Verification items for the finished model (mm, model axes). Face numbers are marked on the shaded views. A direction names the side the tool comes from. Round coordinates to 2 decimals unless told otherwise and drop trailing zeros. Loops run counter-clockwise (first coordinate to the right, second up) from the corner with the lowest first, then second, coordinate; pieces in that order, holes last. Notation, with made-up numbers: M 59.25,6.25 L 66.25,6.25 A17 ccw 66.25,32.25 Z; hole C -31,29 d6. An arc over 180 degrees is marked long. Answer as CSV lines item,"result".
```python
from build123d import *

# Parameters (mm, degrees)
F0_W     = 69
F0_H     = 20
F1_DEPTH = 24
F2_W     = 65
F2_H     = 20
F3_DEPTH = 20
F5_W     = 5
F5_H     = 11
F6_DEPTH = 5


with BuildPart() as f1:
    # F0 (on Front) → F1 (new body)
    with BuildSketch(Plane.XZ):
        with Locations((34.5, -10)):
            Rectangle(F0_W, F0_H)
    extrude(amount=F1_DEPTH)

    # F2 (on Top) → F3 (cut, symmetric)
    with BuildSketch(Plane.XY):
        with Locations((34.5, -12)):
            Rectangle(F2_W, F2_H)
    extrude(amount=F3_DEPTH, both=True, mode=Mode.SUBTRACT)

    # F5 (on offset) → F6 (cut)
    with BuildSketch(Plane(origin=(0, -22, 0), x_dir=(-1, 0, 0), z_dir=(0, 1, 0))):
        with Locations((-22, -10)):
            Rectangle(F5_W, F5_H)
        with Locations((-47, -9.9999997467)):
            Rectangle(F5_W, F5_H)
    extrude(amount=-F6_DEPTH, mode=Mode.SUBTRACT)


solid = f1.part
```
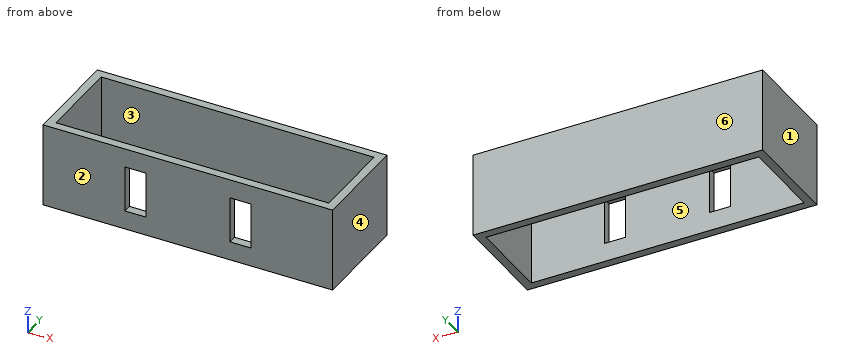
1) Draft check along X on the marked faces 1, 2, 3 and 4. Enter one of: +X half, -X half, draft (parallel to the pull), parting line (faces both ways), or undercut.
Here are the results:
face 1,"-X half"
face 2,"draft"
face 3,"undercut"
face 4,"+X half"
2) Set-up check for the marked faces 5 and 6: record each of +Z, -Z, +X, -X, +Y, -Y from which the full face is reachable in a straight line by a thin tool's end or side.
Here are the results:
face 5,"+Z, -Z"
face 6,"+Z, -Z, +X, -X, +Y"
3) Section check B-B (x = 12). Record the cut outline in (y, z), plus the area to 3 significant figures.
Here are the results:
outline,"M -24,-20 L -22,-20 L -22,0 L -24,0 Z; M -2,-20 L 0,-20 L 0,0 L -2,0 Z"
area,"80.0 mm^2"
4) Section check A-A (z = -11). Record the cut outline in (x, y).
Here are the results:
outline,"M 0,-24 L 19.5,-24 L 19.5,-22 L 2,-22 L 2,-2 L 67,-2 L 67,-22 L 49.5,-22 L 49.5,-24 L 69,-24 L 69,0 L 0,0 Z; M 24.5,-24 L 44.5,-24 L 44.5,-22 L 24.5,-22 Z"
5) Section check C-C (y = -8.25). Record the cut outline in (x, z), plus the area to 3 significant figures.
Here are the results:
outline,"M 0,-20 L 2,-20 L 2,0 L 0,0 Z; M 67,-20 L 69,-20 L 69,0 L 67,0 Z"
area,"80.0 mm^2"
6) Material ranges on probe 1 along X at (y, z) = (-21.5, -2.5); probe 2 along Y at (x, z) = (10, -16.5), recorded low to high.
Here are the results:
probe 1,"x = 0 to 2, 67 to 69"
probe 2,"y = -24 to -22, -2 to 0"
